For this review, take the finished solid that the model builds, in its own axes (mm). Coordinates: 2 decimals unless noted, no trailing zeros. Loops run counter-clockwise (first coordinate to the right, second up) from the corner with the lowest first, then second, coordinate; pieces in that order, holes last. Notation, with made-up numbers: (57.25, -18) - (62.25, -18) arc R33 ccw to (62.25, 12) - close; hole circle Ø3 at (1, -30). An arc over 180 degrees is marked (long way). One line per item, written item: value. Start each with the question number.
1. Take a section at A-A, the plane y = -46.5. State the section outline as (x, z) points.
2. Take a section at C-C, the plane y = -22.5. State the section outline as (x, z) points (3 decimals), and give its area (3 significant figures).
3. Insertion check: pin 1 (0.5 mm diameter, centred on y = -6.5, z = 0.5, fed in from -X); pin 2 (0.8 mm diameter, centred on x = 24.5, z = 1, fed in from -Y); pin 3 (2 mm diameter, centred on x = 2, y = -37.5, fed in from +Z). Each pin has a flat end and moves straight along its axis. Give the tip position at first contact, or say it passes through.
4. Take a section at B-B, the plane x = 29. State the section outline as (y, z) points, and give its area (3 significant figures).
5. To check wall thickness, follow line 1 (Y direction, x = 24, z = 1.3); line 2 (X direction, y = -9.5, z = 1.4); line 3 (Y direction, x = 23.5, z = 0.15). State the ranges of each line that lie inside material, in increasing order. Write a range as from..to.
```python
from build123d import *

# Parameters (mm, degrees)
BOSS_EXTRUDE1_DEPTH = 1.524


with BuildPart() as part:
    # Sketch1 → Boss-Extrude1 (new body)
    with BuildSketch(Plane.XY):
        with BuildLine():
            Line((0, -7.482967549), (0, -5.408604084))
            Line((0, -5.408604084), (0.755403654, -5.408604084))
            Line((0.755403654, -5.408604084), (1.852982052, -6.066483394))
            Line((1.852982052, -6.066483394), (1.852982052, -11.302742268))
            ThreePointArc((1.852982052, -11.302742268), (2.169015936, -14.427077895), (2.651362341, -17.530091345))
            Line((2.651362341, -17.530091345), (3.723597325, -17.530091345))
            Line((3.723597325, -17.530091345), (2.776349352, -18.191976001))
            ThreePointArc((2.776349352, -18.191976001), (3.688558171, -22.143924571), (4.870971382, -26.023605155))
            Line((4.870971382, -26.023605155), (7.391844245, -26.375500189))
            Line((7.391844245, -26.375500189), (5.453722899, -27.64535428))
            ThreePointArc((5.453722899, -27.64535428), (7.526914303, -32.489040294), (10.025271266, -37.127750167))
            Line((10.025271266, -37.127750167), (12.920376423, -36.313179973))
            Line((12.920376423, -36.313179973), (10.828892653, -38.432980418))
            ThreePointArc((10.828892653, -38.432980418), (11.578167935, -39.585157678), (12.354161774, -40.719511876))
            ThreePointArc((12.354161774, -40.719511876), (13.175512701, -41.52681366), (14.230806956, -41.988015948))
            ThreePointArc((14.230806956, -41.988015948), (18.242644995, -43.188625247), (22.0780899, -44.869598037))
            Line((22.0780899, -44.869598037), (24.637655179, -43.847936826))
            Line((24.637655179, -43.847936826), (23.540004987, -45.665371924))
            ThreePointArc((23.540004987, -45.665371924), (28.601111191, -49.226757072), (32.939174514, -53.640311963))
            Line((32.939174514, -53.640311963), (32.658498476, -54.083761868))
            Line((32.658498476, -54.083761868), (30.557652989, -52.629850356))
            Line((30.557652989, -52.629850356), (29.690386669, -53.883016398))
            Line((29.690386669, -53.883016398), (31.842754445, -55.372584435))
            Line((31.842754445, -55.372584435), (31.562078407, -55.81603434))
            ThreePointArc((31.562078407, -55.81603434), (28.171023999, -55.419868819), (25.12237155, -53.883016398))
            Line((25.12237155, -53.883016398), (22.328692601, -53.883016398))
            Line((22.328692601, -53.883016398), (24.149817082, -53.050998637))
            ThreePointArc((24.149817082, -53.050998637), (23.14393246, -51.90329893), (22.328692601, -50.613181701))
            ThreePointArc((22.328692601, -50.613181701), (22.010972611, -50.125385322), (21.609531214, -49.703797722))
            ThreePointArc((21.609531214, -49.703797722), (18.629634099, -47.531264185), (15.315052581, -45.914712875))
            Line((15.315052581, -45.914712875), (12.354161774, -47.327855997))
            Line((12.354161774, -47.327855997), (13.514091924, -45.317136512))
            ThreePointArc((13.514091924, -45.317136512), (12.19400152, -44.990393779), (10.855498604, -44.749957856))
            ThreePointArc((10.855498604, -44.749957856), (9.886950862, -44.4440491), (9.0645671, -43.847936826))
            ThreePointArc((9.0645671, -43.847936826), (8.232032183, -42.969369623), (7.443407514, -42.051183451))
            Line((7.443407514, -42.051183451), (5.583711581, -42.361832951))
            Line((5.583711581, -42.361832951), (6.698610636, -41.092910194))
            ThreePointArc((6.698610636, -41.092910194), (4.549160992, -37.615074341), (3.001052455, -33.831050562))
            Line((3.001052455, -33.831050562), (0.755403654, -33.442087733))
            Line((0.755403654, -33.442087733), (2.67955584, -32.723173894))
            ThreePointArc((2.67955584, -32.723173894), (2.152644596, -30.220357528), (1.886622718, -27.676549835))
            ThreePointArc((1.886622718, -27.676549835), (1.691331674, -26.735134405), (1.223200745, -25.895339764))
            ThreePointArc((1.223200745, -25.895339764), (0.738155144, -25.247811098), (0.2762274, -24.583593236))
            Line((0.2762274, -24.583593236), (-1.923937021, -24.583593236))
            Line((-1.923937021, -24.583593236), (-0.371702809, -23.55840282))
            ThreePointArc((-0.371702809, -23.55840282), (-2.026872481, -20.176102129), (-3.106855858, -16.568723508))
            Line((-3.106855858, -16.568723508), (-5.135572794, -15.725098738))
            Line((-5.135572794, -15.725098738), (-3.3310132, -15.34916898))
            ThreePointArc((-3.3310132, -15.34916898), (-3.571541774, -13.056715378), (-3.580970503, -10.751697242))
            Line((-3.580970503, -10.751697242), (-3.580970503, -6.064514361))
            Line((-3.580970503, -6.064514361), (-2.747975023, -5.406635051))
            Line((-2.747975023, -5.406635051), (-1.524, -5.406635051))
            Line((-1.524, -5.406635051), (-1.524, -7.482967549))
            Line((-1.524, -7.482967549), (0, -7.482967549))
        make_face()
    extrude(amount=BOSS_EXTRUDE1_DEPTH)


solid = part.part
```
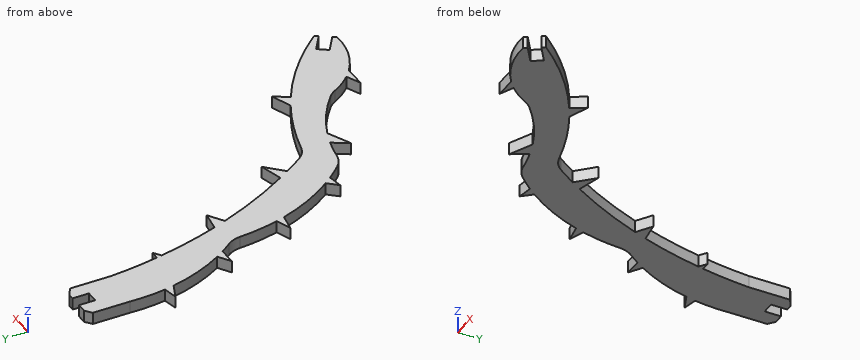
Solutions:
1. outline: (12.83, 0) - (14.09, 0) - (14.09, 1.52) - (12.83, 1.52) - close; (16.69, 0) - (24.91, 0) - (24.91, 1.52) - (16.69, 1.52) - close
2. outline: (-0.965, 0) - (3.785, 0) - (3.785, 1.524) - (-0.965, 1.524) - close
2. area: 7.24 mm2
3. pin 1: x = -3.58
3. pin 2: y = -53.88
3. pin 3: through
4. outline: (-55.63, 0) - (-49.57, 0) - (-49.57, 1.52) - (-55.63, 1.52) - close
4. area: 9.23 mm2
5. line 1: -53.88..-53.12, -52.9..-45.94, -44.9..-44.1
5. line 2: -3.58..1.85
5. line 3: -53.88..-53.35, -52.35..-44.3
